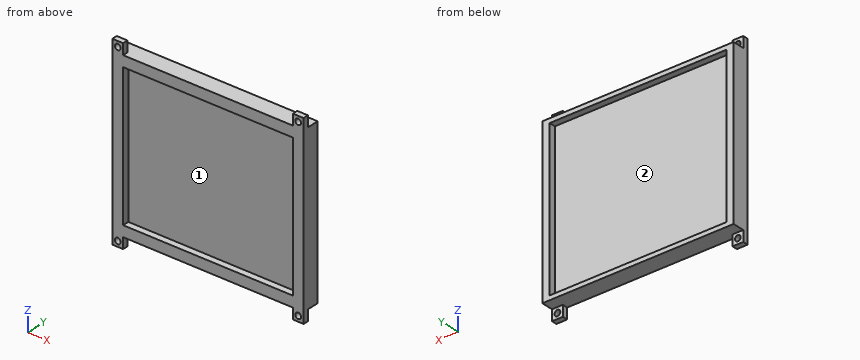
```python
from build123d import *

# Parameters (mm, degrees)
SKETCH1_W           = 112.699999898
SKETCH1_H           = 96.52
BOSS_EXTRUDE1_DEPTH = 10.16
SKETCH2_W           = 104.14
SKETCH2_H           = 91.44
CUT_EXTRUDE1_DEPTH  = 3.81
SKETCH3_W           = 6.35
SKETCH3_H           = 6.35
SKETCH3_R           = 1.7
BOSS_EXTRUDE2_DEPTH = 3.175
SKETCH4_W           = 99.999999898
SKETCH4_H           = 83.82
CUT_EXTRUDE2_DEPTH  = 3.81


with BuildPart() as part:
    # Sketch1 → Boss-Extrude1 (new body)
    with BuildSketch(Plane(origin=(0, 0, 0), x_dir=(1, 0, 0), z_dir=(0, 1, 0))):
        with Locations((56.349999949, 48.26)):
            Rectangle(SKETCH1_W, SKETCH1_H)
    extrude(amount=BOSS_EXTRUDE1_DEPTH)

    # Sketch2 → Cut-Extrude1 (cut)
    with BuildSketch(Plane(origin=(0, 10.16, 0), x_dir=(1, 0, 0), z_dir=(0, 1, 0))):
        with Locations((56.349999949, 48.26)):
            Rectangle(SKETCH2_W, SKETCH2_H)
    extrude(amount=-CUT_EXTRUDE1_DEPTH, mode=Mode.SUBTRACT)

    # Sketch3 → Boss-Extrude2 (add)
    # profile 1 of 4: a face of its own
    with BuildSketch(Plane.XZ):
        with Locations((109.524999898, 3.175)):
            Rectangle(SKETCH3_W, SKETCH3_H)
        with Locations(Location((109.524999898, 3.175, 0), (0, 0, 270))):
            Circle(SKETCH3_R, mode=Mode.SUBTRACT)
    # profile 2 of 4: a face of its own
    with BuildSketch(Plane.XZ):
        with Locations((3.175, 3.175)):
            Rectangle(SKETCH3_W, SKETCH3_H)
        with Locations(Location((3.175, 3.175, 0), (0, 0, 270))):
            Circle(SKETCH3_R, mode=Mode.SUBTRACT)
    # profile 3 of 4: a face of its own
    with BuildSketch(Plane.XZ):
        with Locations((3.175, -99.695)):
            Rectangle(SKETCH3_W, SKETCH3_H)
        with Locations(Location((3.175, -99.695, 0), (0, 0, 270))):
            Circle(SKETCH3_R, mode=Mode.SUBTRACT)
    # profile 4 of 4: a face of its own
    with BuildSketch(Plane.XZ):
        with Locations((109.524999898, -99.695)):
            Rectangle(SKETCH3_W, SKETCH3_H)
        with Locations(Location((109.524999898, -99.695, 0), (0, 0, 270))):
            Circle(SKETCH3_R, mode=Mode.SUBTRACT)
    extrude(amount=-BOSS_EXTRUDE2_DEPTH)

    # Sketch4 → Cut-Extrude2 (cut)
    with BuildSketch(Plane.XZ):
        with Locations((56.349999949, -48.26)):
            Rectangle(SKETCH4_W, SKETCH4_H)
    extrude(amount=-CUT_EXTRUDE2_DEPTH, mode=Mode.SUBTRACT)


solid = part.part
```
For this review, take the finished solid that the model builds, in its own axes (mm). Face numbers are marked on the shaded views. Give positions to 0.01 mm unless a question says otherwise; leave off trailing zeros. Write each loop counter-clockwise with the first axis right and the second up, starting at its lowest first coordinate (ties: lowest second). Pieces come first, ordered by that corner, then holes.
Item 1: Wall thickness on probe 1 along Z at (x, y) = (25.5, 6.5); probe 2 along X at (y, z) = (2.25, -59); probe 3 along X at (y, z) = (7.5, -25): over which ranges is each line inside the solid? List them lowest first.
Item 2: Take a section at C-C (z = -60). Give the boundary of the cut face in (x, y).
Item 3: The part is to be moulded in two halves that separate along Z. For the marked faces 1 and 2, say which applies: +Z half, -Z half, draft (parallel to the pull), parting line (faces both ways), or undercut.
Item 4: Take a section at B-B (y = 8.25). Give the boundary of the cut face in (x, z), and give its area (3 significant figures).
Item 5: Insertion check: P1, Ø4, axis at x = 51, y = 1.5, coming from the +Z side; P2, Ø4, axis at x = 109.525, z = -99.695, coming from the +Y side (3 decimals); P3, Ø2, axis at x = 50, z = -83, coming from the +Y side. Each pin has a flat end and moves straight along its axis. Give the tip position at first contact, or say it passes through.
Item 6: Take a section at A-A (x = 24). Give the boundary of the cut face in (y, z).
Established:
1. probe 1: z = -96.52 to -93.98, -2.54 to 0
1. probe 2: x = 0 to 6.35, 106.35 to 112.7
1. probe 3: x = 0 to 4.28, 108.42 to 112.7
2. outline: (0, 0) - (6.35, 0) - (6.35, 3.81) - (106.35, 3.81) - (106.35, 0) - (112.7, 0) - (112.7, 10.16) - (108.42, 10.16) - (108.42, 6.35) - (4.28, 6.35) - (4.28, 10.16) - (0, 10.16) - close
3. face 1: undercut
3. face 2: undercut
4. outline: (0, -96.52) - (112.7, -96.52) - (112.7, 0) - (0, 0) - close; hole (4.28, -93.98) - (108.42, -93.98) - (108.42, -2.54) - (4.28, -2.54) - close
4. area: 1,360 mm2
5. P1: stops at z = 0
5. P2: stops at y = 3.175
5. P3: stops at y = 6.35
6. outline: (0, -96.52) - (10.16, -96.52) - (10.16, -93.98) - (6.35, -93.98) - (6.35, -2.54) - (10.16, -2.54) - (10.16, 0) - (0, 0) - (0, -6.35) - (3.81, -6.35) - (3.81, -90.17) - (0, -90.17) - close
